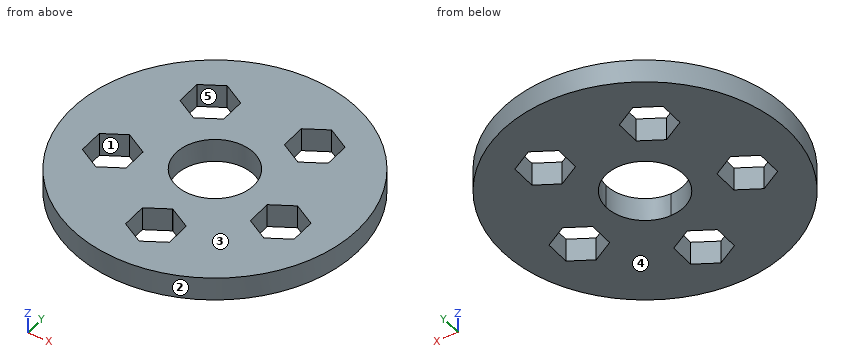
```python
from build123d import *

# Parameters (mm, degrees)
F0_R     = 40.5
F1_DEPTH = 6.66


# Not quite as in the source:
# - a feature names something its author has since deleted; it is built from what else it names


with BuildPart() as f1:
    # F0 (on Top) → F1 (new body)
    with BuildSketch(Plane.XY):
        Circle(F0_R)
        Polygon((-23.7764129074, -14.8754248594), (-29.9684945444, -11.3004248594), (-29.9684945444, -4.1504248594), (-23.7764129074, -0.5754248594), (-17.5843312703, -4.1504248594), (-17.5843312703, -11.3004248594), align=None, mode=Mode.SUBTRACT)
        Polygon((-0.0180177662, -17.8500227021), (0, -17.8603648131), (6.1830530933, -21.4094075078), (6.2010708595, -28.5593848057), (0.0180177662, -32.1499772979), (-6.1830530933, -28.5905924922), (-6.2010708595, -21.4406151943), align=None, mode=Mode.SUBTRACT)
        Polygon((23.7764129074, -0.5754248594), (29.9684945444, -4.1504248594), (29.9684945444, -11.3004248594), (23.7764129074, -14.8754248594), (17.5843312703, -11.3004248594), (17.5843312703, -4.1504248594), align=None, mode=Mode.SUBTRACT)
        Polygon((-14.7765176587, 27.3156769259), (-8.5844360217, 23.7406769259), (-8.5844360217, 16.5906769259), (-14.7765176587, 13.0156769259), (-20.9685992958, 16.5906769259), (-20.9685992958, 23.7406769259), align=None, mode=Mode.SUBTRACT)
        with BuildLine():
            ThreePointArc((0, -11), (-7.7781745931, 7.7781745931), (11, 0))
            ThreePointArc((11, 0), (7.7781745931, -7.7781745931), (0, -11))
        make_face(mode=Mode.SUBTRACT)
        Polygon((14.7765176587, 27.3156769259), (20.9685992958, 23.7406769259), (20.9685992958, 16.5906769259), (14.7765176587, 13.0156769259), (8.5844360217, 16.5906769259), (8.5844360217, 23.7406769259), align=None, mode=Mode.SUBTRACT)
    extrude(amount=F1_DEPTH)


solid = f1.part
```
Geometry check sheet. Reference: the model listing, model coordinates, mm. Face numbers are marked on the shaded views. A direction names the side the tool comes from. Give positions to 0.01 mm unless a question says otherwise; leave off trailing zeros. Loops run counter-clockwise (first coordinate to the right, second up) from the corner with the lowest first, then second, coordinate; pieces in that order, holes last. Notation, with made-up numbers: M 32,65.5 L 82,65.5 A33 ccw 82,96.5 Z; hole C 38.5,-7.75 d9. An arc over 180 degrees is marked long. Write item = value, one per line. Start each with the question number.
1. Tool access check on the marked faces 4 and 5. Record the directions out of +Z, -Z, +X, -X, +Y, -Y that give a thin tool (end or side, any length) a straight path to the whole face; none if there is none.
2. Thickness scan on probe 1 along Y at (x, z) = (0, 4.25); probe 2 along X at (y, z) = (-5, 5); probe 3 along Y at (x, z) = (18, 5). Record the ranges inside material, lowest first.
3. Section check A-A, the plane z = 4.5. Give the number of separate pieces and of enclosed holes in the cut face, plus the area to 3 significant figures.
4. Go/stop test with flat-tipped pins: P1, Ø1, axis at x = -16, z = 2.5, coming from the +Y side; P2, Ø2, axis at y = 22, z = 3.5, coming from the +X side; P3, Ø2, axis at y = 19, z = 3.5, coming from the +X side; P4, Ø4, axis at x = -30, y = -10, coming from the -Z side. Record where each tip stops, or that it passes through.
5. Section check D-D, the plane y = -34. Enter the section's corners in (x, z), plus the area to 3 significant figures.
6. Section check B-B, the plane x = -26. Enter the section's corners in (y, z), plus the area to 3 significant figures.
7. Draft check along X on the marked faces 1, 2 and 3. Enter one of: +X half, -X half, draft (parallel to the pull), parting line (faces both ways), or undercut.
8. Section check C-C, the plane x = -1. Enter the section's corners in (y, z), plus the area to 3 significant figures.
Values follow:
q1.face_4 = -Z, +X, -X, +Y, -Y
q1.face_5 = +Z, -Z
q2.probe_1 = -40.5 to -32.14, -17.86 to -11, 11 to 40.5
q2.probe_2 = -40.19 to -29.97, -17.58 to -9.8, 9.8 to 17.58, 29.97 to 40.19
q2.probe_3 = -36.28 to -11.54, -3.91 to 14.88, 25.45 to 36.28
q3.separate_pieces = 1
q3.enclosed_holes = 6
q3.area = 4,110 mm^2
q4.P1 = 37.42
q4.P2 = 34.63
q4.P3 = 36.28
q4.P4 = 0
q5.outline = M -22.01,0 L 22.01,0 L 22.01,6.66 L -22.01,6.66 Z
q5.area = 293 mm^2
q6.outline = M -31.05,0 L -13.59,0 L -13.59,6.66 L -31.05,6.66 Z; M -1.86,0 L 31.05,0 L 31.05,6.66 L -1.86,6.66 Z
q6.area = 335 mm^2
q7.face_1 = undercut
q7.face_2 = parting line
q7.face_3 = draft
q8.outline = M -40.49,0 L -31.57,0 L -31.57,6.66 L -40.49,6.66 Z; M -18.42,0 L -10.95,0 L -10.95,6.66 L -18.42,6.66 Z; M 10.95,0 L 40.49,0 L 40.49,6.66 L 10.95,6.66 Z
q8.area = 306 mm^2
